Can you work these out from the model? Positions are in its coordinate system, mm. Round coordinates to 2 decimals unless told otherwise and drop trailing zeros. Loops run counter-clockwise (first coordinate to the right, second up) from the corner with the lowest first, then second, coordinate; pieces in that order, holes last. Notation, with made-up numbers: (80.5, 15) -> (92.5, 15) arc R12 ccw to (92.5, 22) -> close; hole circle Ø3 at (-0.5, 18). An arc over 180 degrees is marked (long way). Use a Markdown table: item, result.
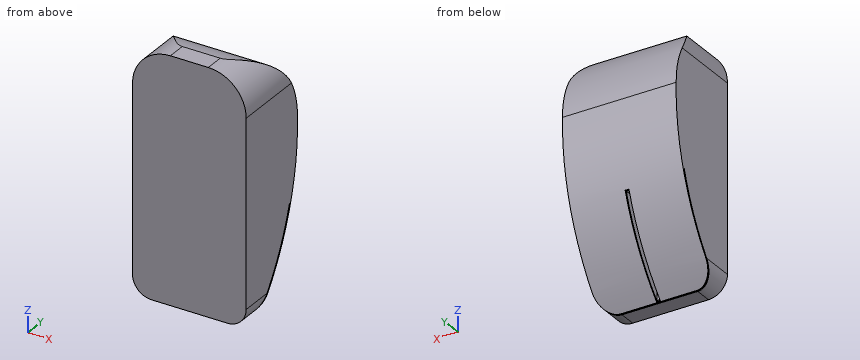
from build123d import *

# Parameters (mm, degrees)
BOSS_EXTRUDE1_DEPTH          = 10
BOSS_EXTRUDE2_DEPTH          = 60
SKETCH1_2_OUTSIDE_W          = 91.554
SKETCH1_2_OUTSIDE_H          = 159.554
CUT_EXTRUDE1_DEPTH           = 60
CUT_EXTRUDE_THIN1_DEPTH      = 148.772850252
CUT_EXTRUDE_THIN1_DEPTH_BACK = 60
SKETCH5_W                    = 2
SKETCH5_H                    = 33
CUT_EXTRUDE2_DEPTH           = 45


with BuildPart() as part:
    # Sketch1 → Boss-Extrude1 (new body)
    with BuildSketch(Plane(origin=(0, 0, 0), x_dir=(1, 0, 0), z_dir=(0, 1, 0))):
        with BuildLine():
            Line((0, 20), (0, 118))
            ThreePointArc((0, 118), (2.928932188, 125.071067812), (10, 128))
            Line((10, 128), (50, 128))
            ThreePointArc((50, 128), (57.071067812, 125.071067812), (60, 118))
            Line((60, 118), (60, 20))
            ThreePointArc((60, 20), (54.142135624, 5.857864376), (40, 0))
            Line((40, 0), (20, 0))
            ThreePointArc((20, 0), (5.857864376, 5.857864376), (0, 20))
        make_face()
    extrude(amount=BOSS_EXTRUDE1_DEPTH)

    # Sketch2 → Boss-Extrude2 (add)
    with BuildSketch(Plane(origin=(0, 0, 0), x_dir=(0, 0, -1), z_dir=(1, 0, 0))):
        with BuildLine():
            Line((0, 10), (128, 10))
            ThreePointArc((128, 10), (87.219557783, 35.085487422), (40, 43))
            ThreePointArc((40, 43), (13.928263114, 33.859681074), (0, 10))
        make_face()
    extrude(amount=BOSS_EXTRUDE2_DEPTH)

    # Sketch1<2> outside → Cut-Extrude1 (cut)
    with BuildSketch(Plane(origin=(0, 0, 0), x_dir=(1, 0, 0), z_dir=(0, 1, 0))):
        with Locations((30, 64)):
            Rectangle(SKETCH1_2_OUTSIDE_W, SKETCH1_2_OUTSIDE_H)
        with BuildLine():
            Line((0, 20), (0, 118))
            ThreePointArc((0, 118), (2.928932188, 125.071067812), (10, 128))
            Line((10, 128), (50, 128))
            ThreePointArc((50, 128), (57.071067812, 125.071067812), (60, 118))
            Line((60, 118), (60, 20))
            ThreePointArc((60, 20), (54.142135624, 5.857864376), (40, 0))
            Line((40, 0), (20, 0))
            ThreePointArc((20, 0), (5.857864376, 5.857864376), (0, 20))
        make_face(mode=Mode.SUBTRACT)
    extrude(amount=CUT_EXTRUDE1_DEPTH, mode=Mode.SUBTRACT)

    # Sketch4 → Cut-Extrude-Thin1 (cut, two sides: drawn at the far end of the back side and taken through both)
    with BuildSketch(Plane.ZY.offset(-CUT_EXTRUDE_THIN1_DEPTH_BACK)):
        with BuildLine():
            ThreePointArc((-81.07900099, 36.207870964), (-106.107453338, 25.30792926), (-128, 9))
            Line((-128, 9), (-128.274111127, 9.291312701))
            ThreePointArc((-128.274111127, 9.291312701), (-106.308105761, 25.653961926), (-81.195672425, 36.590477519))
            Line((-81.195672425, 36.590477519), (-81.07900099, 36.207870964))
        make_face()
    extrude(amount=CUT_EXTRUDE_THIN1_DEPTH + CUT_EXTRUDE_THIN1_DEPTH_BACK, mode=Mode.SUBTRACT)

    # Sketch5 → Cut-Extrude2 (cut)
    with BuildSketch(Plane(origin=(0, 0, -128), x_dir=(-1, 0, 0), z_dir=(0, 0, -1))):
        with Locations((-30, 26.5)):
            Rectangle(SKETCH5_W, SKETCH5_H)
    extrude(amount=-CUT_EXTRUDE2_DEPTH, mode=Mode.SUBTRACT)


solid = part.part
1. I want a section at D-D (y = 20.5). Please give me the cut outline in (x, z).
Answer sheet:
| item | result |
|---|---|
| outline | (0, -114.94) -> (29, -114.94) -> (29, -114.43) -> (0, -114.43) -> close; (0, -113.72) -> (29, -113.72) -> (29, -83) -> (31, -83) -> (31, -113.72) -> (60, -113.72) -> (60, -20) arc R20 ccw to (51.17, -3.41) -> (8.83, -3.41) arc R20 ccw to (0, -20) -> close; (31, -114.94) -> (60, -114.94) -> (60, -114.43) -> (31, -114.43) -> close |
2. Will these pins go through, and if not, where does the flat tip stop? pin 1 Ø1 at (x, y) = (8, 34) entering from +Z; pin 2 Ø10 at (x, z) = (50.5, -52) entering from +Y; pin 3 Ø3 at (x, y) = (18, 19.5) entering from +Z; pin 4 Ø8 at (x, z) = (29.5, -107.5) entering from -Y.
Answer sheet:
| item | result |
|---|---|
| pin 1 | stops at z = -13.5 |
| pin 2 | stops at y = 42.99 |
| pin 3 | stops at z = -2.3 |
| pin 4 | stops at y = 0 |
3. I want a section at A-A (y = 27.5). Please give me the cut outline in (x, z), plus the area to 3 significant figures.
Answer sheet:
| item | result |
|---|---|
| outline | (0, -103.7) -> (29, -103.7) -> (29, -103.01) -> (0, -103.01) -> close; (0, -102.16) -> (29, -102.16) -> (29, -83) -> (31, -83) -> (31, -102.16) -> (60, -102.16) -> (60, -20) arc R20 ccw to (55.82, -7.76) -> (4.18, -7.76) arc R20 ccw to (0, -20) -> close; (31, -103.7) -> (60, -103.7) -> (60, -103.01) -> (31, -103.01) -> close |
| area | 5,630 mm² |
4. I need wall thicknesses on line 1 (X direction, y = 29, z = -94.5); line 2 (Z direction, x = 20.5, y = 23.5); line 3 (Y direction, x = 33, z = -45). Which ranges of each line are inside material? Lowest first, please.
Answer sheet:
| item | result |
|---|---|
| line 1 | x = 0 to 29, 31 to 60 |
| line 2 | z = -110.44 to -109.88, -109.12 to -5.03 |
| line 3 | y = 0 to 43.03 |
5. I want a section at C-C (x = 24). Please give me the cut outline in (y, z), plus the area to 3 significant figures.
Answer sheet:
| item | result |
|---|---|
| outline | (0, -128) -> (9, -128) arc R119.21 ccw to (36.21, -81.08) -> (36.59, -81.2) arc R119.61 cw to (9.55, -128) -> (10, -128) arc R125 ccw to (43, -40) arc R40 ccw to (10, 0) -> (0, 0) -> close |
| area | 4,290 mm² |
6. I want a section at B-B (z = -114). Please give me the cut outline in (x, y), plus the area to 3 significant figures.
Answer sheet:
| item | result |
|---|---|
| outline | (0, 0) -> (60, 0) -> (60, 20.31) -> (31, 20.31) -> (31, 10) -> (29, 10) -> (29, 20.31) -> (0, 20.31) -> close; (0, 20.79) -> (29, 20.79) -> (29, 21.15) -> (0, 21.15) -> close; (31, 20.79) -> (60, 20.79) -> (60, 21.15) -> (31, 21.15) -> close |
| area | 1,220 mm² |
